from build123d import *

# Parameters (mm, degrees)
BOSS_EXTRUDE1_DEPTH         = 6.0452
FILLET1_R                   = 20
TAP_DRILL_FOR_M3X0_5_TAP1_D = 2.5
CUT_EXTRUDE1_REACH          = 31.611
SKETCH6_R                   = 1.5875
SKETCH6_R_2                 = 1.4605
CUT_EXTRUDE2_START          = -6.0452
CUT_EXTRUDE2_DEPTH          = 6.0452


with BuildPart() as part:
    # Sketch1 → Boss-Extrude1 (new body)
    with BuildSketch(Plane(origin=(0, 0, 0), x_dir=(1, 0, 0), z_dir=(0, 1, 0))):
        with BuildLine():
            Line((6.34428877, -4), (24, -4))
            ThreePointArc((24, -4), (28, 0), (24, 4))
            Line((24, 4), (6.34428877, 4))
            ThreePointArc((6.34428877, 4), (-7.5, 0), (6.34428877, -4))
        make_face()
    extrude(amount=BOSS_EXTRUDE1_DEPTH)

    # Fillet1
    fillet1_edges = [part.edges().sort_by_distance(p)[0] for p in [
        (6.34428877, 3.0226, -4),
        (6.34428877, 3.0226, 4),
    ]]
    fillet(fillet1_edges, radius=FILLET1_R)

    # Tap Drill for M3x0.5 Tap1 (through all)
    with Locations(Plane(origin=(0, 6.0452, 0), x_dir=(1, 0, 0), z_dir=(0, 1, 0))):
        with Locations((19.301, 0), (24, 0)):
            Hole(TAP_DRILL_FOR_M3X0_5_TAP1_D / 2)

    # Sketch6 → Cut-Extrude1 (cut, up to next)
    with BuildSketch(Plane(origin=(0, 6.0452, 0), x_dir=(1, 0, 0), z_dir=(0, 1, 0)), mode=Mode.PRIVATE) as cut_extrude1_sk1:
        with Locations(Location((0, 0, 0), (0, 0, 270))):
            Circle(SKETCH6_R)
    cut_extrude1_tool1 = extrude(cut_extrude1_sk1.sketch, amount=-CUT_EXTRUDE1_REACH, mode=Mode.PRIVATE) & part.part
    # Sketch6 → Cut-Extrude1 (cut, up to next)
    with BuildSketch(Plane(origin=(0, 6.0452, 0), x_dir=(1, 0, 0), z_dir=(0, 1, 0)), mode=Mode.PRIVATE) as cut_extrude1_sk2:
        with Locations(Location((8.731458325, 0, 0), (0, 0, 270))):
            Circle(SKETCH6_R_2)
    cut_extrude1_tool2 = extrude(cut_extrude1_sk2.sketch, amount=-CUT_EXTRUDE1_REACH, mode=Mode.PRIVATE) & part.part
    add(cut_extrude1_tool1.solids().sort_by_distance((0, 6.0452, 0))[0], mode=Mode.SUBTRACT)
    add(cut_extrude1_tool2.solids().sort_by_distance((8.731458, 6.0452, 0))[0], mode=Mode.SUBTRACT)

    # Sketch7 → Cut-Extrude2 (cut)
    with BuildSketch(Plane(origin=(0, 6.0452, 0), x_dir=(1, 0, 0), z_dir=(0, 1, 0)).offset(CUT_EXTRUDE2_START)):
        with BuildLine():
            Line((7.449638443, 0.6999986), (-7.467262012, 0.6999986))
            ThreePointArc((-7.467262012, 0.6999986), (-7.5, -1.406e-06), (-7.46726175, -0.7000014))
            Line((-7.46726175, -0.7000014), (7.449639972, -0.7000014))
            ThreePointArc((7.449639972, -0.7000014), (7.270958325, -1.595e-06), (7.449638443, 0.6999986))
        make_face()
    extrude(amount=CUT_EXTRUDE2_DEPTH, mode=Mode.SUBTRACT)


solid = part.part
Verification items for the finished model (mm, model axes). A direction names the side the tool comes from. Give positions to 0.01 mm unless a question says otherwise; leave off trailing zeros. Order: outer loops, then holes, each group sorted by start corner. A loop starts at its lowest first (then second) coordinate and runs counter-clockwise, first axis right, second up. Notation, with made-up numbers: M 0.25,-28 L 27.25,-28 A18 cw 27.25,-22 Z; hole C 25.25,35 d9. An arc over 180 degrees is marked long. Answer as a JSON object with one key per item and string values. Group by question number.
1) Cross-section at C-C (x = 4). Enter the section's corners in (y, z), then the cut area to 3 significant figures.
2) Cross-section at D-D (x = 15.5). Enter the section's corners in (y, z), then the cut area to 3 significant figures.
3) Cross-section at B-B (y = 2.75). Give the number of separate pieces and of enclosed holes in the cut face, then the cut area to 3 significant figures.
4) Mould release check, pull along Z, two halves, no side actions. Record for faces 1 (the face through (8.45, 3.06, -4.63)), 2 (the face through (4, 3, 0.7)), 3 (the face through (8.45, 3.06, 4.63)): released by +Z, released by -Z, zero draft, split by the parting line, or undercut.
5) Access from +Z, -Z, +X, -X, +Y, -Y to the whole of each face (thin tool, end or side, straight path). Record for faces 4 (the face through (-0.025, 3.065, 1.587)), 5 (the face through (-4, 3, 0.7)), 6 (the face through (19, 3, 4)), 7 (the face through (19, 3, -4)).
6) Depth check by flat-ended pin: pin 1 Ø1.8 at (x, y) = (-5, 2) entering from +Z; pin 2 Ø1.8 at (x, y) = (-5, 3.5) entering from -Z; pin 3 Ø2 at (y, z) = (4.5, 5.5) entering from -X. Enter the tip coordinate at first touch or a pass-through.
7) Cross-section at A-A (z = 0). Enter the section's corners in (x, y).
8) Scan lines: line 1 along X through (y, z) = (0.5, 0.5); line 2 along X through (y, z) = (5, -0.75); line 3 along Z through (x, y) = (24, 1.75). Record each from-to range of solid material in increasing order. Write a range as [from, to].
Result sheet:
{
 "1": {"outline": "M 0,-6.36 L 6.05,-6.36 L 6.05,-0.7 L 0,-0.7 Z; M 0,0.7 L 6.05,0.7 L 6.05,6.36 L 0,6.36 Z", "area": "68.4 mm2"},
 "2": {"outline": "M 0,-4 L 6.05,-4 L 6.05,4 L 0,4 Z", "area": "48.4 mm2"},
 "3": {"separate pieces": "1", "enclosed holes": "2", "area": "304 mm2"},
 "4": {"face 1": "released by -Z", "face 2": "undercut", "face 3": "released by +Z"},
 "5": {"face 4": "+Y, -Y", "face 5": "-X, +Y, -Y", "face 6": "+Z, +X, +Y, -Y", "face 7": "-Z, +X, +Y, -Y"},
 "6": {"pin 1": "stops at z = 6.28", "pin 2": "stops at z = -6.28", "pin 3": "stops at x = -6"},
 "7": {"outline": "M 10.19,0 L 18.05,0 L 18.05,6.05 L 10.19,6.05 Z; M 20.55,0 L 22.75,0 L 22.75,6.05 L 20.55,6.05 Z; M 25.25,0 L 28,0 L 28,6.05 L 25.25,6.05 Z"},
 "8": {"line 1": "x = [10.1, 18.16], [20.45, 22.85], [25.15, 27.97]", "line 2": "x = [-7.46, -1.4], [1.4, 7.48], [9.98, 18.3], [20.3, 23], [25, 27.93]", "line 3": "z = [-4, -1.25], [1.25, 4]"}
}
